Here's how the part is built. I have some questions about the finished solid (model axes, mm). Face numbers are marked on the shaded views. A direction names the side the tool comes from. Give positions to 0.01 mm unless a question says otherwise; leave off trailing zeros. Order: outer loops, then holes, each group sorted by start corner. A loop starts at its lowest first (then second) coordinate and runs counter-clockwise, first axis right, second up.
from build123d import *

# Parameters (mm, degrees)
SKETCH1_R           = 50
BOSS_EXTRUDE1_DEPTH = 30
SKETCH2_R           = 15
BOSS_EXTRUDE2_DEPTH = 12.5


with BuildPart() as part:
    # Sketch1 → Boss-Extrude1 (new body)
    with BuildSketch(Plane(origin=(0, 0, 0), x_dir=(1, 0, 0), z_dir=(0, 1, 0))):
        with Locations(Location((0, 0, 0), (0, 0, 270))):
            Circle(SKETCH1_R)
    extrude(amount=BOSS_EXTRUDE1_DEPTH)

    # Sketch2 → Boss-Extrude2 (add, symmetric)
    with BuildSketch(Plane(origin=(0, 0, 0), x_dir=(0, 0, -1), z_dir=(1, 0, 0))):
        with BuildLine():
            Line((-25, 70), (-25, 30))
            Line((-25, 30), (25, 30))
            Line((25, 30), (25, 70))
            ThreePointArc((25, 70), (0, 95), (-25, 70))
        make_face()
        with Locations((0, 70)):
            Circle(SKETCH2_R, mode=Mode.SUBTRACT)
    extrude(amount=BOSS_EXTRUDE2_DEPTH, both=True)


solid = part.part
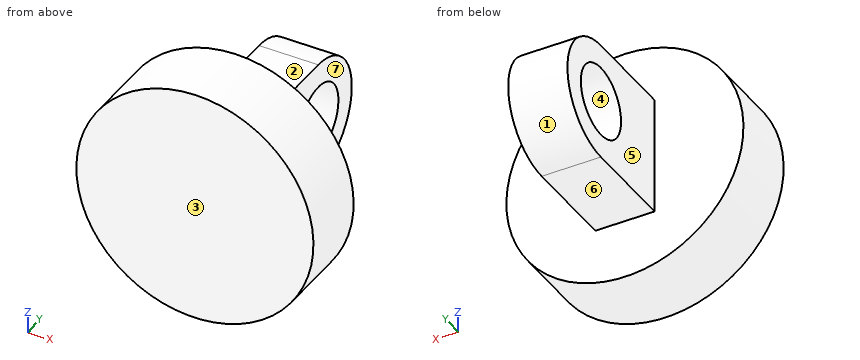
Q1. If we section it at A-A on z = 0: List the corners of the cut face in (x, y) for me, plus the area to 4 significant figures.
Filled sheet:
outline: (-50, 0) - (50, 0) - (50, 30) - (12.5, 30) - (12.5, 55) - (-12.5, 55) - (-12.5, 30) - (-50, 30) - close; (-12.5, 85) - (12.5, 85) - (12.5, 95) - (-12.5, 95) - close
area: 3,875 mm2
Q2. For the marked faces 5, 6 and 7, which set-ups out of +Z, -Z, +X, -X, +Y, -Y let a thin tool reach every point of the face, with its end or its side?
Filled sheet:
face 5: +Z, -Z, -X, +Y
face 6: -Z, +X, -X, +Y
face 7: +Z, -Z, +X, +Y
Q3. Thinking about a two-plate mould opening in Y: for the marked faces 1, 2, 3 and 4, which applies, released by +Y, released by -Y, zero draft, split by the parting line, or undercut?
Filled sheet:
face 1: released by +Y
face 2: zero draft
face 3: released by -Y
face 4: undercut
Q4. If we section it at C-C on x = 0: List the corners of the cut face in (y, z) for me.
Filled sheet:
outline: (0, -50) - (30, -50) - (30, -25) - (70, -25) arc R25 ccw to (70, 25) - (30, 25) - (30, 50) - (0, 50) - close; hole circle Ø30 at (70, 0)
Q5. I need wall thicknesses on L1, parallel to Y at x = -5, z = 0; L2, parallel to Y at x = -13, z = 4; L3, parallel to X at y = 78, z = 15.5. Which ranges of each line are inside material? Lowest first, please.
Filled sheet:
L1: y = 0 to 55, 85 to 95
L2: y = 0 to 30
L3: x = -12.5 to 12.5
Q6. I'm going to push flat-ended pins straight in: P1, Ø5, axis at y = 55.5, z = -25, coming from the -X side; P2, Ø6, axis at y = 32, z = 36.5, coming from the -X side; P3, Ø2, axis at y = 44.5, z = -2.5, coming from the +X side; P4, Ø18, axis at y = 70, z = 0, coming from the +X side. Where does each tip first touch, or does it pass through?
Filled sheet:
P1: stops at x = -12.5
P2: stops at x = -36.41
P3: stops at x = 12.5
P4: passes through
Q7. If we section it at D-D on y = 43.5: List the corners of the cut face in (x, z) for me, plus the area to 3 significant figures.
Filled sheet:
outline: (-12.5, -25) - (12.5, -25) - (12.5, 25) - (-12.5, 25) - close
area: 1,250 mm2
Q8. If we section it at B-B on y = 72.5: List the corners of the cut face in (x, z) for me, plus the area to 3 significant figures.
Filled sheet:
outline: (-12.5, -24.87) - (12.5, -24.87) - (12.5, -14.79) - (-12.5, -14.79) - close; (-12.5, 14.79) - (12.5, 14.79) - (12.5, 24.87) - (-12.5, 24.87) - close
area: 504 mm2
